Could you check a few things on this drawing? It's one solid part, dimensions in mm from its lowest x, y, z. Give positions to 0.01 mm unless a question says otherwise; leave off trailing zeros. Loops run counter-clockwise (first coordinate to the right, second up) from the corner with the lowest first, then second, coordinate; pieces in that order, holes last. Notation, with made-up numbers: (-9.75, -22.5) -> (-3.75, -22.5) arc R14 cw to (-3.75, -15.5) -> close; hole circle Ø7 at (40, -39.75). An arc over 180 degrees is marked (long way). Use CSV: the item, a comma, the result in double quotes.
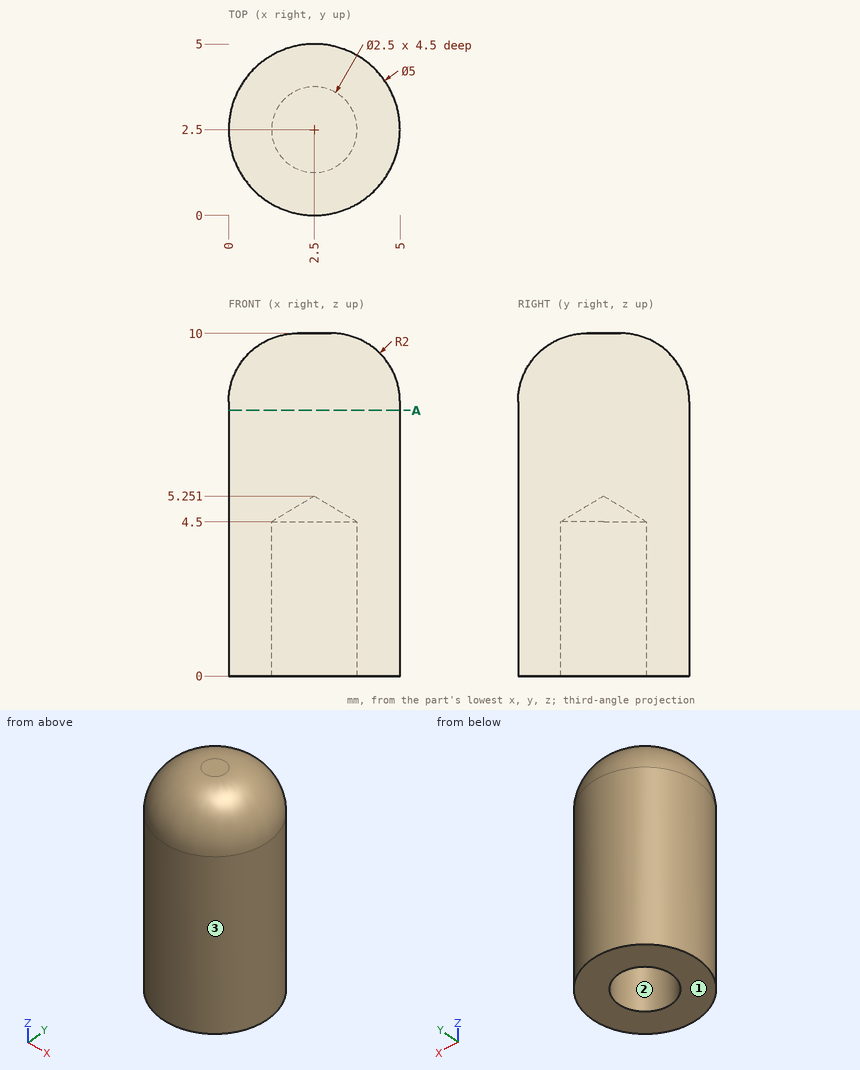
(1) If we section it at A-A, the plane z = 7.75: Write out the boundary of the cut face in (x, y).
Answer sheet:
outline,"circle Ø5 at (2.5, 2.5)"
(2) If I drill on L1, parallel to Y at x = 2.5, z = 1.55; L2, parallel to Y at x = 3.35, z = 3.5; L3, parallel to X at y = 2.6, z = 7, over which ranges is the centre line in solid material (lowest first)? Write a range as from..to.
Answer sheet:
L1,"y = 0..1.25, 3.75..5"
L2,"y = 0.15..1.58, 3.42..4.85"
L3,"x = 0..5"
(3) We'd pull the mould along Y, two halves only. Please class the marked faces 1, 2 and 3: released by +Y, released by -Y, zero draft, split by the parting line, or undercut.
Answer sheet:
face 1,"zero draft"
face 2,"undercut"
face 3,"split by the parting line"
(4) Will these pins go through, and if not, where does the flat tip stop? pin 1 Ø1.5 at (y, z) = (1.5, 9) entering from +X; pin 2 Ø2 at (x, z) = (4, 9) entering from -Y.
Answer sheet:
pin 1,"stops at x = 4.9"
pin 2,"stops at y = 0.14"
